from build123d import *

# Parameters (mm, degrees)
SKETCH_W        = 32
SKETCH_H        = 32
PAD_DEPTH       = 10
SKETCH001_R     = 1.5
PAD001_DEPTH    = 15
SKETCH002_R     = 2
SKETCH002_W     = 15
SKETCH002_H     = 15
PAD002_DEPTH    = 12
SKETCH003_W     = 32
SKETCH003_H     = 10
PAD003_DEPTH    = 40
SKETCH004_W     = 32
SKETCH004_H     = 10
PAD004_DEPTH    = 40
SKETCH006_W     = 20
SKETCH006_H     = 25
POCKET_DEPTH    = 10.001
SKETCH005_W     = 20
SKETCH005_H     = 25
POCKET001_DEPTH = 10.001


with BuildPart() as part:
    # Sketch → Pad (new body)
    with BuildSketch(Plane.XY):
        with Locations((16, 16)):
            Rectangle(SKETCH_W, SKETCH_H)
    extrude(amount=PAD_DEPTH)

    # Sketch001 (on Face6 of Pad) → Pad001 (join)
    with BuildSketch(Plane.XY.offset(10)):
        with Locations((4, 29.5)):
            Circle(SKETCH001_R)
        with Locations((28, 29.5)):
            Circle(SKETCH001_R)
        with Locations((4, 2.5)):
            Circle(SKETCH001_R)
        with Locations((28, 2.5)):
            Circle(SKETCH001_R)
    extrude(amount=PAD001_DEPTH)

    # Sketch002 (on Face5 of Pad001) → Pad002 (join)
    with BuildSketch(Plane.XY.offset(10)):
        with Locations((4, 2.5)):
            Circle(SKETCH002_R)
        with Locations((28, 2.5)):
            Circle(SKETCH002_R)
        with Locations((4, 29.5)):
            Circle(SKETCH002_R)
        with Locations((28, 29.5)):
            Circle(SKETCH002_R)
        with Locations((16, 16)):
            Rectangle(SKETCH002_W, SKETCH002_H)
    extrude(amount=PAD002_DEPTH)

    # Sketch003 (on Face1 of Pad002) → Pad003 (join)
    with BuildSketch(Plane.XZ):
        with Locations((16, 5)):
            Rectangle(SKETCH003_W, SKETCH003_H)
    extrude(amount=PAD003_DEPTH)

    # Sketch004 (on Face2 of Pad003) → Pad004 (join)
    with BuildSketch(Plane(origin=(0, 32, 0), x_dir=(-1, 0, 0), z_dir=(0, 1, 0))):
        with Locations((-16, 5)):
            Rectangle(SKETCH004_W, SKETCH004_H)
    extrude(amount=PAD004_DEPTH)

    # Sketch006 (on Face6 of Pad004) → Pocket (cut, through all)
    with BuildSketch(Plane.XY.offset(10)):
        with Locations((16, 52)):
            Rectangle(SKETCH006_W, SKETCH006_H)
    extrude(amount=-POCKET_DEPTH, mode=Mode.SUBTRACT)

    # Sketch005 (on Face10 of Pad004) → Pocket001 (cut, through all)
    with BuildSketch(Plane.XY.offset(10)):
        with Locations((16, -20)):
            Rectangle(SKETCH005_W, SKETCH005_H)
    extrude(amount=-POCKET001_DEPTH, mode=Mode.SUBTRACT)


solid = part.part
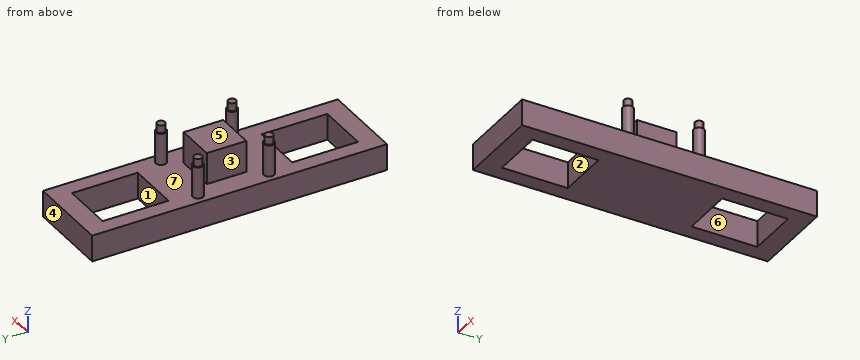
Design review of the part built by this model. Coordinates are the model's own, in mm. Face numbers are marked on the shaded views. A direction names the side the tool comes from. Round coordinates to 2 decimals unless told otherwise and drop trailing zeros. Loops run counter-clockwise (first coordinate to the right, second up) from the corner with the lowest first, then second, coordinate; pieces in that order, holes last. Notation, with made-up numbers: (64, 34) -> (109, 34) arc R32 ccw to (109, 60) -> close; hole circle Ø9 at (47, 3). An arc over 180 degrees is marked (long way). Use one line per item in the form item = value. Start each with the question number.
Q1. Machinability: for the marked faces 5, 6 and 7, which of the approach directions +Z, -Z, +X, -X, +Y, -Y give a long, thin tool a straight path to every point of the face, cutting with its end or side? Answer none if there is none.
Q2. We need section B-B on z = 7.25. Give the boundary of the cut face in (x, y), then the cut area to 3 significant figures.
Q3. We need section C-C on x = 11. Give the boundary of the cut face in (y, z), then the cut area to 3 significant figures.
Q4. We need section A-A on y = 57. Give the boundary of the cut face in (x, z).
Q5. Wall thickness on line 1 along Y through (x, z) = (17.5, 8.5); line 2 along X through (y, z) = (-18.5, 7.5); line 3 along Z through (x, y) = (16, 27.5): over which ranges is each line inside the solid? List them lowest first. Write a range as [from, to].
Q6. For pin 1 Ø16.5 at (x, y) = (16, 19) entering from +Z; pin 2 Ø9.5 at (x, z) = (13, 17) entering from +Y; pin 3 Ø13 at (x, z) = (13.5, 18.5) entering from -Y, all flat-tipped, find the tip position at first contact; note any pin that passes through.
Q7. We need section D-D on z = 15. Give the boundary of the cut face in (x, y), then the cut area to 3 significant figures.
Q8. Draft analysis for pull direction X (two halves, no side actions). For the marked faces 1, 2, 3 and 4, state which applies: +X half, -X half, draft (parallel to the pull), parting line (faces both ways), or undercut.
Calculated:
q1.face_5 = +Z, +X, -X, +Y, -Y
q1.face_6 = +Z, -Z
q1.face_7 = +Z
q2.outline = (0, -40) -> (32, -40) -> (32, 72) -> (0, 72) -> close; hole (6, -32.5) -> (26, -32.5) -> (26, -7.5) -> (6, -7.5) -> close; hole (6, 39.5) -> (26, 39.5) -> (26, 64.5) -> (6, 64.5) -> close
q2.area = 2,580 mm²
q3.outline = (-40, 0) -> (-32.5, 0) -> (-32.5, 10) -> (-40, 10) -> close; (-7.5, 0) -> (39.5, 0) -> (39.5, 10) -> (23.5, 10) -> (23.5, 22) -> (8.5, 22) -> (8.5, 10) -> (-7.5, 10) -> close; (64.5, 0) -> (72, 0) -> (72, 10) -> (64.5, 10) -> close
q3.area = 800 mm²
q4.outline = (0, 0) -> (6, 0) -> (6, 10) -> (0, 10) -> close; (26, 0) -> (32, 0) -> (32, 10) -> (26, 10) -> close
q5.line_1 = [-40, -32.5], [-7.5, 39.5], [64.5, 72]
q5.line_2 = [0, 6], [26, 32]
q5.line_3 = [0, 10]
q6.pin_1 = 22
q6.pin_2 = 23.5
q6.pin_3 = 8.5
q7.outline = circle Ø4 at (4, 2.5); circle Ø4 at (4, 29.5); (8.5, 8.5) -> (23.5, 8.5) -> (23.5, 23.5) -> (8.5, 23.5) -> close; circle Ø4 at (28, 2.5); circle Ø4 at (28, 29.5)
q7.area = 275 mm²
q8.face_1 = undercut
q8.face_2 = undercut
q8.face_3 = -X half
q8.face_4 = draft
